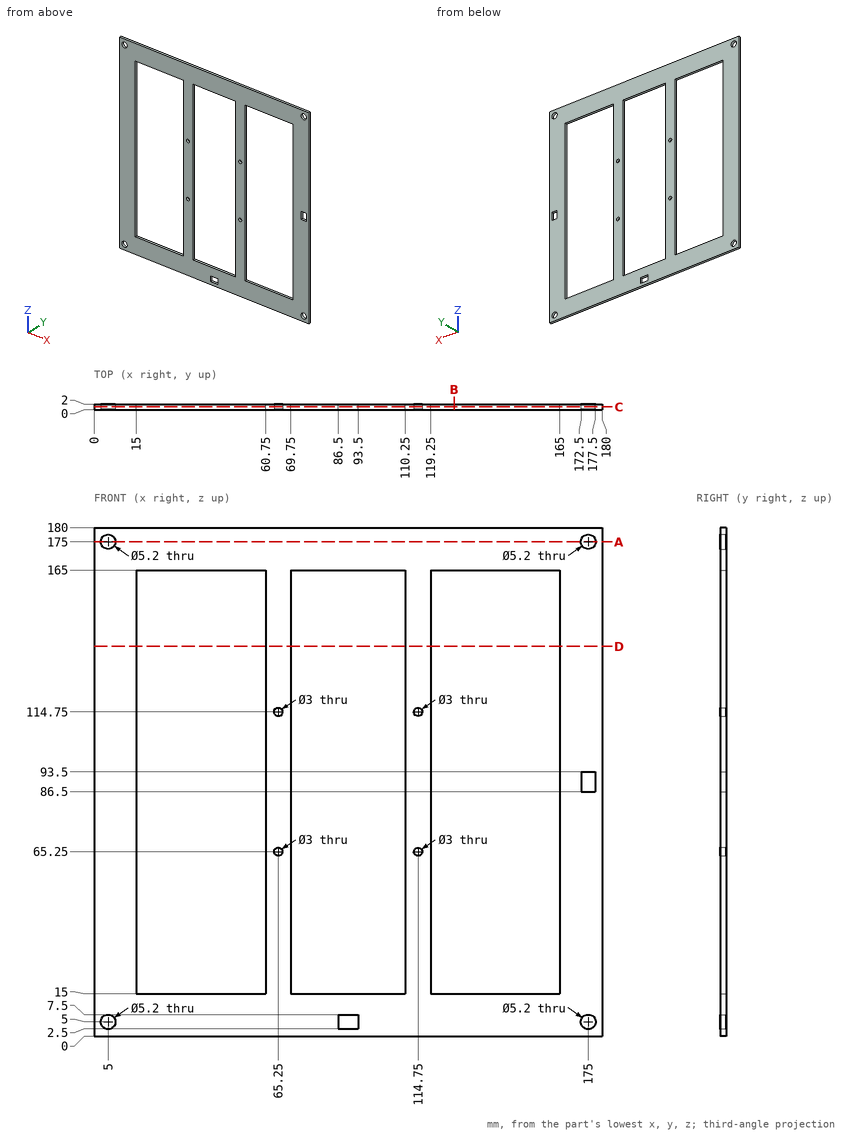
Job drawing, mm, ordinate dimensions from the low corner. One solid piece. Give positions to 0.01 mm unless a question says otherwise; leave off trailing zeros. Order: outer loops, then holes, each group sorted by start corner. A loop starts at its lowest first (then second) coordinate and runs counter-clockwise, first axis right, second up. Notation, with made-up numbers: (-17.5, 22) - (19.5, 22) arc R32 ccw to (19.5, 56) - close; hole circle Ø10 at (19, 53.5). An arc over 180 degrees is marked (long way). Answer in a Markdown table with one row per item.
1. Probe probe 1 along Z at (x, y) = (114.75, 0.8); probe 2 along X at (y, z) = (1.1, 26); probe 3 along X at (y, z) = (0.8, 87). List the from-to ranges inside material, lowest first. Write a range as [from, to].
Data:
| item | result |
|---|---|
| probe 1 | z = [0, 63.75], [66.75, 113.25], [116.25, 180] |
| probe 2 | x = [0, 15], [60.75, 69.75], [110.25, 119.25], [165, 180] |
| probe 3 | x = [0, 15], [60.75, 69.75], [110.25, 119.25], [165, 172.5], [177.5, 180] |
2. Saw through at B-B, the plane x = 127.5. Give the cut face in (y, z).
Data:
| item | result |
|---|---|
| outline | (0, 0) - (2, 0) - (2, 15) - (0, 15) - close; (0, 165) - (2, 165) - (2, 180) - (0, 180) - close |
3. Saw through at A-A, the plane z = 175. Give the cut face in (x, y), plus the area to 3 significant figures.
Data:
| item | result |
|---|---|
| outline | (0, 0) - (2.4, 0) - (2.4, 2) - (0, 2) - close; (7.6, 0) - (172.4, 0) - (172.4, 2) - (7.6, 2) - close; (177.6, 0) - (180, 0) - (180, 2) - (177.6, 2) - close |
| area | 339 mm² |
4. Saw through at C-C, the plane y = 1. Count the separate pieces of the cut face and the enclosed holes in it, plus the area to 3 significant figures.
Data:
| item | result |
|---|---|
| separate pieces | 1 |
| enclosed holes | 13 |
| area | 12,400 mm² |
5. Saw through at D-D, the plane z = 138. Give the cut face in (x, y), plus the area to 3 significant figures.
Data:
| item | result |
|---|---|
| outline | (0, 0) - (15, 0) - (15, 2) - (0, 2) - close; (60.75, 0) - (69.75, 0) - (69.75, 2) - (60.75, 2) - close; (110.25, 0) - (119.25, 0) - (119.25, 2) - (110.25, 2) - close; (165, 0) - (180, 0) - (180, 2) - (165, 2) - close |
| area | 96.0 mm² |
